The listing builds one solid part. Answer for the finished solid, in the listing's coordinates (mm). Face numbers are marked on the shaded views. Give positions to 0.01 mm unless a question says otherwise; leave off trailing zeros. Loops run counter-clockwise (first coordinate to the right, second up) from the corner with the lowest first, then second, coordinate; pieces in that order, holes last. Notation, with made-up numbers: (76, -4.75) - (81, -4.75) arc R17 cw to (81, 4.25) - close; hole circle Ø5 at (-1, -23). An arc over 180 degrees is marked (long way). Write each question's results on one line, items separated by ' | '.
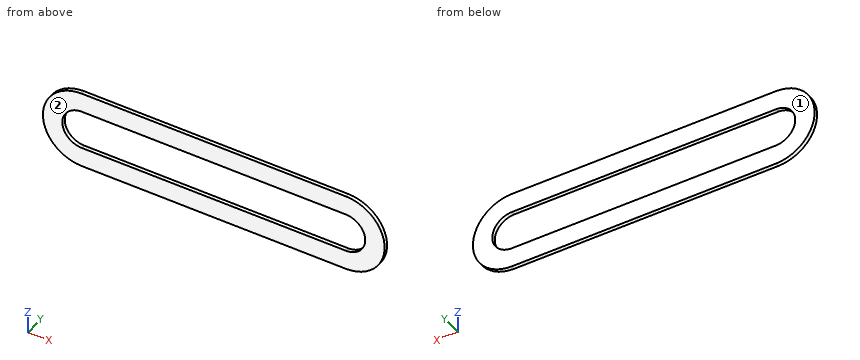
from build123d import *

# Parameters (mm, degrees)
BOSS_EXTRUDE1_DEPTH = 0.5


with BuildPart() as part:
    # Sketch1 → Boss-Extrude1 (new body)
    with BuildSketch(Plane(origin=(0, 0, 0), x_dir=(1, 0, 0), z_dir=(0, 1, 0))):
        with BuildLine():
            ThreePointArc((0, -5), (5, 0), (0, 5))
            Line((0, 5), (-34, 5))
            ThreePointArc((-34, 5), (-39, 0), (-34, -5))
            Line((-34, -5), (0, -5))
        make_face()
        with BuildLine():
            ThreePointArc((-34, -2.5), (-36.5, 0), (-34, 2.5))
            Line((-34, 2.5), (0, 2.5))
            ThreePointArc((0, 2.5), (2.5, 0), (0, -2.5))
            Line((0, -2.5), (-34, -2.5))
        make_face(mode=Mode.SUBTRACT)
    extrude(amount=BOSS_EXTRUDE1_DEPTH)


solid = part.part
Item 1: For a pull along Y with two mould halves and no side action, classify the marked faces 1 and 2 as released by +Y, released by -Y, zero draft, split by the parting line, or undercut.
Values found:
face 1: released by +Y | face 2: released by -Y
Item 2: A cutting plane is placed at B-B, the plane x = -27. Determine the outline of the cut face in (y, z), plus the area to 3 significant figures.
Values found:
outline: (0, -5) - (0.5, -5) - (0.5, -2.5) - (0, -2.5) - close; (0, 2.5) - (0.5, 2.5) - (0.5, 5) - (0, 5) - close | area: 2.50 mm²
Item 3: Find the intervals of material crossed by line 1 along Z through (x, y) = (-3.5, 0.3); line 2 along X through (y, z) = (0.35, 0.5); line 3 along Z through (x, y) = (-35, 0.3), in increasing order. Write a range as [from, to].
Values found:
line 1: z = [-5, -2.5], [2.5, 5] | line 2: x = [-38.97, -36.45], [2.45, 4.97] | line 3: z = [-4.9, -2.29], [2.29, 4.9]
Item 4: A cutting plane is placed at C-C, the plane y = 0.15. Determine the outline of the cut face in (x, z), plus the area to 3 significant figures.
Values found:
outline: (-34, -5) - (0, -5) arc R5 ccw to (0, 5) - (-34, 5) arc R5 ccw to start; hole (-34, -2.5) - (0, -2.5) arc R2.5 ccw to (0, 2.5) - (-34, 2.5) arc R2.5 ccw to start | area: 229 mm²
Item 5: A cutting plane is placed at A-A, the plane z = 0. Determine the outline of the cut face in (x, y).
Values found:
outline: (-39, 0) - (-36.5, 0) - (-36.5, 0.5) - (-39, 0.5) - close; (2.5, 0) - (5, 0) - (5, 0.5) - (2.5, 0.5) - close
Item 6: A cutting plane is placed at D-D, the plane z = 4. Determine the outline of the cut face in (x, y).
Values found:
outline: (-37, 0) - (3, 0) - (3, 0.5) - (-37, 0.5) - close
